Build history of the part. All positions in model axes, mm. A direction names the side the tool comes from. Round coordinates to 2 decimals unless told otherwise and drop trailing zeros. Order: outer loops, then holes, each group sorted by start corner. A loop starts at its lowest first (then second) coordinate and runs counter-clockwise, first axis right, second up. Notation, with made-up numbers: (2.25, 80) -> (58.25, 80) arc R7 ccw to (58.25, 90) -> close; hole circle Ø6 at (-40, 8). An arc over 180 degrees is marked (long way). Use a Markdown table: item, result. Add a question column.
Item 1: Pin check, flat tips, straight feed: pin 1 (18.5 mm diameter, centred on y = 36, z = 0, fed in from +X); pin 2 (19 mm diameter, centred on x = -13.5, z = 24, fed in from +Y); pin 3 (3 mm diameter, centred on x = -36, z = 22, fed in from -Y); pin 4 (8 mm diameter, centred on x = -57, z = 3, fed in from -Y). Stop position of each tip, or through.
Item 2: Two-plate mould, pull along Z, no slides. Class faces 1 (the face through (61, 16, 0)), 2 (the face through (61, 52, 0)), 3 (the face through (-17, 15, -32)): released by +Z, released by -Z, zero draft, split by the parting line, or undercut.
Item 3: Slice it at B-B, the plane z = 0. Give the cut face in (x, y), plus the area to 3 significant figures.
Item 4: Slice it at D-D, the plane x = 58.5. Give the cut face in (y, z), plus the area to 3 significant figures.
Item 5: Slice it at C-C, the plane y = 26.5. Give the cut face in (x, z), plus the area to 3 significant figures.
Item 6: 3-axis set-ups, long thin cutter, end or side, ignore diameter. For faces 4 (the face through (61.15, 30.07, -20.42)), 5 (the face through (1, 7, -12)), 6 (the face through (-34.66, 5.07, 19.89)), 7 (the face through (61.154, 43.932, 1.041)): which of +Z, -Z, +X, -X, +Y, -Y reach the whole face in a straight line?
Item 7: Probe L1, parallel to X at y = 6.75, z = 22; L2, parallel to Z at x = 34, y = 4.5; L3, parallel to Z at x = 33, y = 9.5. List the from-to ranges inside material, lowest first.
Item 8: Slice it at A-A, the plane x = 10. Give the cut face in (y, z), plus the area to 3 significant figures.
from build123d import *

# Parameters (mm, degrees)
SKETCH1_W                 = 144
SKETCH1_H                 = 64
BOSS_EXTRUDE1_DEPTH       = 16
BOSS_EXTRUDE2_DEPTH       = 64
SKETCH3_R                 = 8
BOSS_EXTRUDE3_DEPTH       = 22
FILLET1_R                 = 3
CUT_EXTRUDE1_DEPTH        = 157.409718368
M6X1_0_TAPPED_HOLE1_D     = 5
M6X1_0_TAPPED_HOLE1_DEPTH = 10
M6X1_0_TAPPED_HOLE1_TIP   = 1.443375673


with BuildPart() as part:
    # Sketch1 → Boss-Extrude1 (new body)
    with BuildSketch(Plane(origin=(0, 0, 0), x_dir=(1, 0, 0), z_dir=(0, 1, 0))):
        Rectangle(SKETCH1_W, SKETCH1_H)
    extrude(amount=BOSS_EXTRUDE1_DEPTH)

    # Sketch2 → Boss-Extrude2 (add)
    with BuildSketch(Plane.XY.offset(32)):
        Polygon((-46, 16), (-46, 52), (-56, 52), (-72, 36), (-72, 16), align=None)
    extrude(amount=-BOSS_EXTRUDE2_DEPTH)

    # Sketch3 → Boss-Extrude3 (add)
    with BuildSketch(Plane(origin=(72, 0, 0), x_dir=(0, 0, -1), z_dir=(1, 0, 0))):
        with BuildLine():
            Line((-14.500924593, 42.761892188), (-26.980199866, 16))
            Line((-26.980199866, 16), (26.980199866, 16))
            Line((26.980199866, 16), (14.500924593, 42.761892188))
            ThreePointArc((14.500924593, 42.761892188), (0, 52), (-14.500924593, 42.761892188))
        make_face()
        with Locations((0, 36)):
            Circle(SKETCH3_R, mode=Mode.SUBTRACT)
    extrude(amount=-BOSS_EXTRUDE3_DEPTH)

    # Fillet1
    fillet1_edges = [part.edges().sort_by_distance(p)[0] for p in [
        (61, 16, -26.980199866),
        (61, 16, 26.980199866),
    ]]
    fillet(fillet1_edges, radius=FILLET1_R)

    # Sketch4 → Cut-Extrude1 (cut, through all)
    with BuildSketch(Plane(origin=(72, 0, 0), x_dir=(0, 0, -1), z_dir=(1, 0, 0))):
        Polygon((-16, 0), (-16, 7), (-8, 7), (-8, 16), (8, 16), (8, 7), (16, 7), (16, 0), align=None)
    extrude(amount=-CUT_EXTRUDE1_DEPTH, mode=Mode.SUBTRACT)

    # M6x1.0 Tapped Hole1
    with Locations(Plane(origin=(0, 0, 0), x_dir=(-1, 0, 0), z_dir=(0, -1, 0))):
        with Locations((-34, -22), (36, -22), (36, 22), (-34, 22)):
            Hole(M6X1_0_TAPPED_HOLE1_D / 2, depth=M6X1_0_TAPPED_HOLE1_DEPTH)
            with Locations((0, 0, -(M6X1_0_TAPPED_HOLE1_DEPTH + M6X1_0_TAPPED_HOLE1_TIP / 2))):  # 120° drill point
                Cone(0, M6X1_0_TAPPED_HOLE1_D / 2, M6X1_0_TAPPED_HOLE1_TIP, mode=Mode.SUBTRACT)


solid = part.part
Check sheet entries:
| question | item | result |
|---|---|---|
| 1 | pin 1 | x = 72 |
| 1 | pin 2 | y = 16 |
| 1 | pin 3 | y = 10.58 |
| 1 | pin 4 | y = 16 |
| 2 | face 1 | undercut |
| 2 | face 2 | split by the parting line |
| 2 | face 3 | released by -Z |
| 3 | outline | (-72, 16) -> (-46, 16) -> (-46, 52) -> (-56, 52) -> (-72, 36) -> close; (50, 16) -> (72, 16) -> (72, 28) -> (50, 28) -> close; (50, 44) -> (72, 44) -> (72, 52) -> (50, 52) -> close |
| 3 | area | 1,250 mm2 |
| 4 | outline | (0, -32) -> (16, -32) -> (16, -28.89) arc R3 cw to (17.73, -26.17) -> (42.76, -14.5) arc R16 ccw to (42.76, 14.5) -> (17.73, 26.17) arc R3 cw to (16, 28.89) -> (16, 32) -> (0, 32) -> (0, 16) -> (7, 16) -> (7, 8) -> (16, 8) -> (16, -8) -> (7, -8) -> (7, -16) -> (0, -16) -> close; hole circle Ø16 at (36, 0) |
| 4 | area | 1,760 mm2 |
| 5 | outline | (-72, -32) -> (-46, -32) -> (-46, 32) -> (-72, 32) -> close; (50, -22.08) -> (72, -22.08) -> (72, 22.08) -> (50, 22.08) -> close |
| 5 | area | 2,640 mm2 |
| 6 | face 4 | -Z, +X, +Y |
| 6 | face 5 | +X, -X, -Y |
| 6 | face 6 | -Y |
| 6 | face 7 | +X |
| 7 | L1 | -72 to -38.5, -33.5 to 31.5, 36.5 to 72 |
| 7 | L2 | -32 to -24.5, -19.5 to -16, 16 to 19.5, 24.5 to 32 |
| 7 | L3 | -32 to -24.29, -19.71 to -8, 8 to 19.71, 24.29 to 32 |
| 8 | outline | (0, -32) -> (16, -32) -> (16, -8) -> (7, -8) -> (7, -16) -> (0, -16) -> close; (0, 16) -> (7, 16) -> (7, 8) -> (16, 8) -> (16, 32) -> (0, 32) -> close |
| 8 | area | 656 mm2 |
